from build123d import *

# Parameters (mm, degrees)
F1_DEPTH = 6


with BuildPart() as f1:
    # F0 (on Top) → F1 (new body)
    with BuildSketch(Plane.XY):
        with BuildLine():
            ThreePointArc((-37.1493010532, -12.3887201771), (-39.7850652933, 2.6112798229), (-37.1493010532, 17.6112798229))
            Line((-37.1493010532, 17.6112798229), (-65.7850652933, 17.6112798229))
            Line((-65.7850652933, 17.6112798229), (-65.7850652933, -12.3887201771))
            Line((-65.7850652933, -12.3887201771), (-37.1493010532, -12.3887201771))
        make_face()
        with BuildLine():
            ThreePointArc((-4.798943482, -12.3887201771), (-13.2850652933, 2.6112798229), (-4.798943482, 17.6112798229))
            Line((-4.798943482, 17.6112798229), (-37.1493010532, 17.6112798229))
            ThreePointArc((-37.1493010532, 17.6112798229), (-39.7850652933, 2.6112798229), (-37.1493010532, -12.3887201771))
            Line((-37.1493010532, -12.3887201771), (-4.798943482, -12.3887201771))
        make_face()
        with BuildLine():
            ThreePointArc((13.2288128953, 17.6112798229), (19.4463638632, 11.2283307018), (21.7149347067, 2.6112798229))
            ThreePointArc((21.7149347067, 2.6112798229), (19.4463638632, -6.005771056), (13.2288128953, -12.3887201771))
            Line((13.2288128953, -12.3887201771), (45.5791704666, -12.3887201771))
            ThreePointArc((45.5791704666, -12.3887201771), (47.5509842119, -5.0036274833), (48.2149347067, 2.6112798229))
            ThreePointArc((48.2149347067, 2.6112798229), (47.5509842119, 10.2261871291), (45.5791704666, 17.6112798229))
            Line((45.5791704666, 17.6112798229), (13.2288128953, 17.6112798229))
        make_face()
        with BuildLine():
            Line((74.2149347067, 17.6112798229), (45.5791704666, 17.6112798229))
            ThreePointArc((45.5791704666, 17.6112798229), (47.5509842119, 10.2261871291), (48.2149347067, 2.6112798229))
            ThreePointArc((48.2149347067, 2.6112798229), (47.5509842119, -5.0036274833), (45.5791704666, -12.3887201771))
            Line((45.5791704666, -12.3887201771), (74.2149347067, -12.3887201771))
            Line((74.2149347067, -12.3887201771), (74.2149347067, 17.6112798229))
        make_face()
        with BuildLine():
            ThreePointArc((-4.798943482, 17.6112798229), (4.2149347067, 20.1112798229), (13.2288128953, 17.6112798229))
            Line((13.2288128953, 17.6112798229), (45.5791704666, 17.6112798229))
            ThreePointArc((45.5791704666, 17.6112798229), (35.703112855, 33.3439112901), (20.2149347067, 43.5990828867))
            Line((20.2149347067, 43.5990828867), (20.2149347067, 37.6344849233))
            Line((20.2149347067, 37.6344849233), (-11.7850652933, 37.6344849233))
            Line((-11.7850652933, 37.6344849233), (-11.7850652933, 43.5990828867))
            ThreePointArc((-11.7850652933, 43.5990828867), (-27.2732434416, 33.3439112901), (-37.1493010532, 17.6112798229))
            Line((-37.1493010532, 17.6112798229), (-4.798943482, 17.6112798229))
        make_face()
        with BuildLine():
            Line((45.5791704666, -12.3887201771), (13.2288128953, -12.3887201771))
            ThreePointArc((13.2288128953, -12.3887201771), (4.2149347067, -14.8887201771), (-4.798943482, -12.3887201771))
            Line((-4.798943482, -12.3887201771), (-37.1493010532, -12.3887201771))
            ThreePointArc((-37.1493010532, -12.3887201771), (4.2149347067, -41.3887201771), (45.5791704666, -12.3887201771))
        make_face()
    extrude(amount=F1_DEPTH)


solid = f1.part
CAD build for the part. Positions are in the model's coordinates, mm. A direction names the side the tool comes from. Give positions to 0.01 mm unless a question says otherwise; leave off trailing zeros. Loops run counter-clockwise (first coordinate to the right, second up) from the corner with the lowest first, then second, coordinate; pieces in that order, holes last. Notation, with made-up numbers: M 3.25,86 L 10.25,86 A30 ccw 10.25,117 Z; hole C 19.25,78 d11. An arc over 180 degrees is marked long. One line per question, with ' | ' between items. Start each with the question number.
1. Saw through at A-A on z = 3.2. Give the cut face in (x, y).
2. Saw through at D-D on y = 14.5. Give the cut face in (x, z), plus the area to 3 significant figures.
3. Saw through at C-C on x = 59. Give the cut face in (y, z).
4. Two-plate mould, pull along X, no slides. Class faces 4 (the face through (60, 17.611, 3)), 5 (the face through (-65.785, 3, 3)), 6 (the face through (-11.785, 41, 3)), 7 (the face through (74.215, 2, 3)): pulls with the +X half, pulls with the -X half, needs draft (parallel to the pull), parting line crosses it, or undercut.
5. 3-axis set-ups, long thin cutter, end or side, ignore diameter. For faces 1 (the face through (-52, -12.389, 3)), 2 (the face through (4, 37.634, 3)), 3 (the face through (60, -12.389, 3)): which of +Z, -Z, +X, -X, +Y, -Y reach the whole face in a straight line?
6. Probe L1, parallel to X at y = -3.5, z = 0.45; L2, parallel to X at y = 14, z = 3.65; L3, parallel to Y at x = 17.5, z = 5.1. List the from-to ranges inside material, lowest first. Write a range as from..to.
7. Saw through at B-B on y = -9.5. Give the cut face in (x, z).
8. Flat gauge pins, fed straight in: pin 1 (2 mm diameter, centred on x = 47, z = 4.5, fed in from -Y); pin 2 (1.8 mm diameter, centred on x = 56, z = 3, fed in from +Y); pin 3 (3 mm diameter, centred on y = 39, z = 3.5, fed in from -X). Where does each tip first touch, or does it go through?
Result sheet:
1) outline: M -65.79,-12.39 L -37.15,-12.39 A44 ccw 45.58,-12.39 L 74.21,-12.39 L 74.21,17.61 L 45.58,17.61 A44 ccw 20.21,43.6 L 20.21,37.63 L -11.79,37.63 L -11.79,43.6 A44 ccw -37.15,17.61 L -65.79,17.61 Z; hole C 4.21,2.61 d35
2) outline: M -65.79,0 L -8.63,0 L -8.63,6 L -65.79,6 Z; M 17.06,0 L 74.21,0 L 74.21,6 L 17.06,6 Z | area: 686 mm^2
3) outline: M -12.39,0 L 17.61,0 L 17.61,6 L -12.39,6 Z
4) face 4: needs draft | face 5: pulls with the -X half | face 6: undercut | face 7: pulls with the +X half
5) face 1: +Z, -Z, -X, -Y | face 2: +Z, -Z, +Y | face 3: +Z, -Z, +X, -Y
6) L1: x = -65.79..-12.18, 20.61..74.21 | L2: x = -65.79..-9.07, 17.5..74.21 | L3: y = -39.34..-8.78, 14..37.63
7) outline: M -65.79,0 L -8.42,0 L -8.42,6 L -65.79,6 Z; M 16.85,0 L 74.21,0 L 74.21,6 L 16.85,6 Z
8) pin 1: stops at y = -12.39 | pin 2: stops at y = 17.61 | pin 3: stops at x = -22.6
